Answer from the drawing. Dimensions are ordinates in mm from the lowest x, y and z of the part. A direction names the side the tool comes from. Coordinates: 2 decimals unless noted, no trailing zeros. Write each loop counter-clockwise with the first axis right and the second up, starting at its lowest first coordinate (ties: lowest second). Pieces come first, ordered by that corner, then holes.
(1) The part is cut by section C-C, the plane z = 65. Determine the outline of the cut face in (x, y), and give its area (3 significant figures).
(2) The part is cut by section D-D, the plane x = 6. Determine the outline of the cut face in (y, z).
(3) The part is cut by section B-B, the plane y = 31. Determine the outline of the cut face in (x, z), and give its area (3 significant figures).
(4) Straight lines are drawn through the part: line 1 along Z through (x, y) = (2, 7); line 2 along Y through (x, z) = (24, 52.75); line 3 along X through (y, z) = (1.5, 65). For each, find the intervals that lie inside material, in ascending order.
(5) Given pin 1 (3 mm diameter, centred on x = 26, z = 65, fed in from +Y) (3 decimals); pin 2 (14 mm diameter, centred on x = 25, y = 22.5, fed in from -Z); pin 3 (5 mm diameter, centred on y = 9, z = 19, fed in from +X); pin 4 (3 mm diameter, centred on x = 18, z = 47, fed in from +Y), each flat-ended and moving along its own axis, determine where each tip first touches the part or whether it passes through.
(6) Which of the six approach directions +Z, -Z, +X, -X, +Y, -Y give full straight-line access (tool end or side, diameter ignored) to the marked faces 1, 2 and 3?
(7) The part is cut by section A-A, the plane y = 6.5. Determine the outline of the cut face in (x, z), and give its area (3 significant figures).
(8) Determine the mould class of the marked faces 4, 5, 6 and 7 for opening direction Z: pulls with the +Z half, pulls with the -Z half, needs draft (parallel to the pull), parting line crosses it, or undercut.
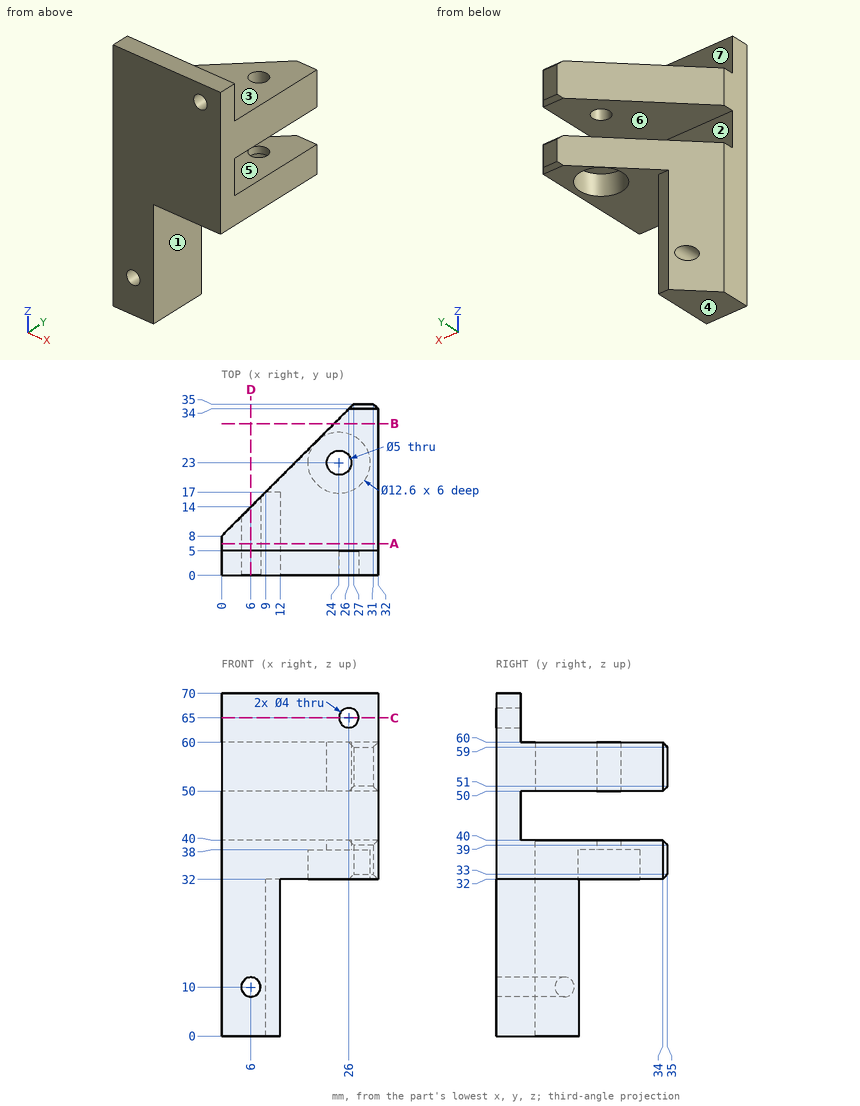
Computed:
1. outline: (0, 0) - (24, 0) - (24, 5) - (0, 5) - close; (28, 0) - (32, 0) - (32, 5) - (28, 5) - close
1. area: 140 mm2
2. outline: (0, 0) - (14, 0) - (14, 8) - (0, 8) - close; (0, 12) - (14, 12) - (14, 40) - (5, 40) - (5, 50) - (14, 50) - (14, 60) - (5, 60) - (5, 70) - (0, 70) - close
3. outline: (23, 32) - (32, 32) - (32, 40) - (23, 40) - close; (23, 50) - (32, 50) - (32, 60) - (23, 60) - close
3. area: 162 mm2
4. line 1: z = 0 to 40, 50 to 60
4. line 2: y = 0 to 20.5, 25.5 to 32
4. line 3: x = 0 to 24, 28 to 32
5. pin 1: passes through
5. pin 2: stops at z = 32
5. pin 3: stops at x = 12
5. pin 4: stops at y = 5
6. face 1: -Z, +X, +Y, -Y
6. face 2: +X, -X, +Y
6. face 3: +Z, +X, -X, +Y
7. outline: (0, 0) - (12, 0) - (12, 32) - (32, 32) - (32, 40) - (0, 40) - close; (0, 50) - (32, 50) - (32, 60) - (0, 60) - close; hole circle Ø4 at (6, 10)
7. area: 947 mm2
8. face 4: pulls with the -Z half
8. face 5: undercut
8. face 6: undercut
8. face 7: needs draft
